Source: three-view drawing plus pictorial views. Frame: mm from the lowest corner of the part. A direction names the side the tool comes from. Coordinates: 2 decimals unless noted, no trailing zeros. Write each loop counter-clockwise with the first axis right and the second up, starting at its lowest first coordinate (ties: lowest second). Pieces come first, ordered by that corner, then holes. Notation, with made-up numbers: (48, 15.5) - (60, 15.5) arc R26 cw to (60, 40.5) - close; hole circle Ø7 at (26, -34). An arc over 180 degrees is marked (long way). Put each result on its own line as item: value.
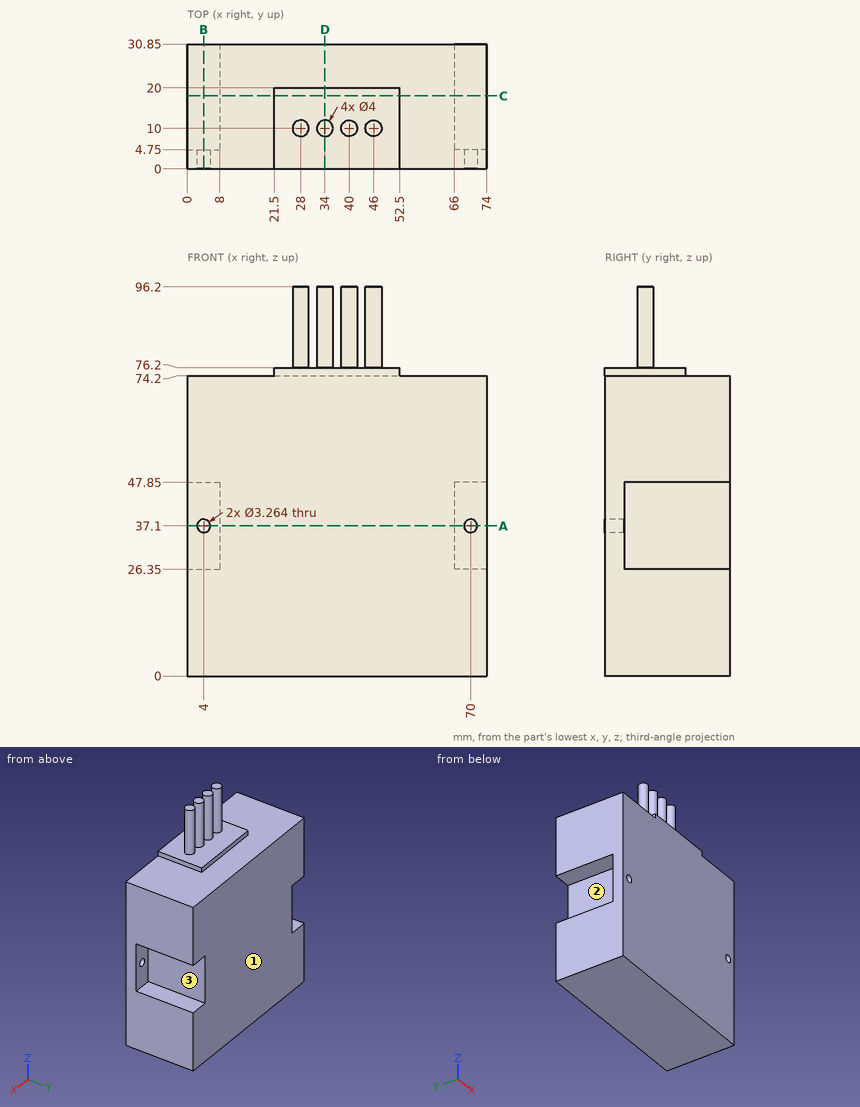
1. Section query D-D (x = 34). Return loops of the section in (y, z), then the cut area to 3 significant figures.
Answer below:
outline: (0, 0) - (30.85, 0) - (30.85, 74.2) - (20, 74.2) - (20, 76.2) - (12, 76.2) - (12, 96.2) - (8, 96.2) - (8, 76.2) - (0, 76.2) - close
area: 2,410 mm²
2. Section query B-B (x = 4). Return loops of the section in (y, z).
Answer below:
outline: (0, 0) - (30.85, 0) - (30.85, 26.35) - (4.75, 26.35) - (4.75, 35.47) - (0, 35.47) - close; (0, 38.73) - (4.75, 38.73) - (4.75, 47.85) - (30.85, 47.85) - (30.85, 74.2) - (0, 74.2) - close
3. Pin query (flat end, axial travel): pin 1 Ø12 at (y, z) = (9, 33.5) entering from +X; pin 2 Ø6.5 at (y, z) = (17, 38.5) entering from -X; pin 3 Ø0.6 at (x, z) = (34.5, 75.5) entering from +Y; pin 4 Ø6 at (y, z) = (13, 32) entering from +X. Return the tip coordinate at first contact, or that it passes through.
Answer below:
pin 1: stops at x = 74
pin 2: stops at x = 8
pin 3: stops at y = 20
pin 4: stops at x = 66
4. Section query C-C (y = 18). Return loops of the section in (x, z), then the cut area to 3 significant figures.
Answer below:
outline: (0, 0) - (74, 0) - (74, 26.35) - (66, 26.35) - (66, 47.85) - (74, 47.85) - (74, 74.2) - (52.5, 74.2) - (52.5, 76.2) - (21.5, 76.2) - (21.5, 74.2) - (0, 74.2) - (0, 47.85) - (8, 47.85) - (8, 26.35) - (0, 26.35) - close
area: 5,210 mm²
5. Ray query, probe 1 along X at (y, z) = (3, 37); probe 2 along Z at (x, y) = (67, 13); probe 3 along Z at (x, y) = (70, 3). Return the intervals inside material, ascending. Write a range as from..to.
Answer below:
probe 1: x = 0..2.37, 5.63..68.37, 71.63..74
probe 2: z = 0..26.35, 47.85..74.2
probe 3: z = 0..35.47, 38.73..74.2
6. Section query A-A (z = 37.1). Return loops of the section in (x, y).
Answer below:
outline: (0, 0) - (2.37, 0) - (2.37, 4.75) - (0, 4.75) - close; (5.63, 0) - (68.37, 0) - (68.37, 4.75) - (66, 4.75) - (66, 30.85) - (8, 30.85) - (8, 4.75) - (5.63, 4.75) - close; (71.63, 0) - (74, 0) - (74, 4.75) - (71.63, 4.75) - close
7. Set-up query: the marked faces 1, 2 and 3. Return all of +Z, -Z, +X, -X, +Y, -Y with unobstructed straight access to the full face (end or side cutting, diameter ignored); none if empty.
Answer below:
face 1: +Z, -Z, +X, -X, +Y
face 2: -X, +Y
face 3: +X, +Y
